The model under review builds one solid part; all positions refer to its coordinate system, in mm. A direction names the side the tool comes from. Coordinates: 2 decimals unless noted, no trailing zeros. Order: outer loops, then holes, each group sorted by start corner. A loop starts at its lowest first (then second) coordinate and runs counter-clockwise, first axis right, second up. Notation, with made-up numbers: M 71.25,13.5 L 95.25,13.5 A30 cw 95.25,46.5 Z; hole C -32.75,37.25 d10. An arc over 180 degrees is marked long. Answer in a Markdown table with one row per item.
Autodesk Inventor part; units mm, degrees
ref_plane "YZ Plane" through (0, 0, 0) normal (1, 0, 0) x (0, 1, 0)
ref_plane "XZ Plane" through (0, 0, 0) normal (0, 1, 0) x (-1, 0, 0)
ref_plane "XY Plane" through (0, 0, 0) normal (0, 0, 1) x (1, 0, 0)
sketch "Sketch1" plane through (0, 0, 0) normal (0, 0, 1) x (1, 0, 0)
  circle A0 centre (0, -12.7) radius 3.175
  circle A1 centre (12.7, 0) radius 3.175
  circle A2 centre (0, 12.7) radius 3.175
  circle A3 centre (-12.7, 0) radius 3.175
  line L0 (25.4, 57.15) -> (-25.4, 57.15)
  line L1 (-25.4, 57.15) -> (-25.4, -57.15)
  line L2 (-25.4, -57.15) -> (25.4, -57.15)
  line L3 (25.4, -57.15) -> (25.4, 57.15)
  point P0 (0, 0)
  dimension "d1" = 6.35
  dimension "d2" = 12.7
  dimension "d5" = 360
  dimension "d13" = 25.4
  dimension "d14" = 57.15
  dimension "d15" = 57.15
  dimension "d16" = 25.4
extrude "Extrusion3" add sketch "Sketch1" along normal blind 6.35
sketch "Sketch3" plane through (0, 0, 6.35) normal (0, 0, 1) x (1, 0, 0)
  line L0 (25.4, 57.15) -> (-25.4, 57.15)
  line L1 (25.4, 57.15) -> (25.4, 50.8)
  line L2 (25.4, -57.15) -> (25.4, 57.15)
  line L3 (25.4, 50.8) -> (-25.4, 50.8)
  line L4 (-25.4, 57.15) -> (-25.4, -57.15)
  line L5 (-25.4, 57.15) -> (25.4, 57.15)
  line L6 (-25.4, -57.15) -> (25.4, -57.15)
  line L7 (25.4, -57.15) -> (25.4, -50.8)
  line L8 (25.4, -50.8) -> (-25.4, -50.8)
  line L9 (-25.4, -50.8) -> (-25.4, -57.15)
  line L10 (-25.4, -57.15) -> (25.4, -57.15)
  point P0 (0, 0)
  dimension "d19" = 6.35
  dimension "d20" = 6.35
extrude "Extrusion4" add sketch "Sketch3" along normal blind 50.8 contours L1 L3 L4 L0 | L2 L6 L4 L8
fillet "Fillet1" radius 3.175 8 edges at (25.4, 53.975, 57.15) (25.4, -53.975, 57.15) (-25.4, -53.975, 57.15) (-25.4, 53.975, 57.15) (0, -57.15, 0) (0, 57.15, 0) (0, -50.8, 6.35) (0, 50.8, 6.35)
sketch "Sketch6" plane through (0, 0, 6.35) normal (0, 0, 1) x (1, 0, 0)
  circle A0 centre (0, 0) radius 3.175
  dimension "d50" = 6.35
extrude "Extrusion6" add sketch "Sketch6" along normal blind 12.7
sketch "Sketch7" plane through (-25.4, 57.15, 3.175) normal (0, 1, 0) x (1, 0, 0)
  line L0 (47.625, -53.975) -> (3.175, -53.975)
  line L1 (0, 0) -> (0, -50.8)
  line L2 (47.625, -53.975) -> (3.175, -53.975)
  line L3 (38.1, -53.975) -> (38.1, -60.325)
  line L4 (12.7, -60.325) -> (12.7, -53.975)
  line L5 (38.1, -60.325) -> (31.75, -60.325)
  line L6 (19.05, -60.325) -> (12.7, -60.325)
  line L7 (38.1, -53.975) -> (12.7, -53.975)
  arc A0 (31.75, -60.325) -> (25.4, -53.975) centre (25.4, -60.325) ccw
  arc A1 (25.4, -53.975) -> (19.05, -60.325) centre (25.4, -60.325) ccw
  point P0 (25.4, 3.175)
  dimension "d57" = 38.1
  dimension "d58" = 12.7
  dimension "d59" = 6.35
  dimension "d60" = 6.35
  dimension "d66" = 6.35
  dimension "d67" = 25.4
  dimension "d68" = 6.35
  dimension "d69" = 25.4
extrude "Extrusion7" add sketch "Sketch7" against normal blind 6.35
sketch "Sketch8" plane through (-25.4, -57.15, 3.175) normal (0, -1, 0) x (1, 0, 0)
  line L0 (12.7, 53.975) -> (12.7, 60.325)
  line L1 (12.7, 53.975) -> (12.7, 60.325)
  line L2 (38.1, 60.325) -> (38.1, 53.975)
  line L3 (38.1, 60.325) -> (38.1, 53.975)
  line L4 (38.1, 53.975) -> (25.4, 53.975)
  line L5 (47.625, 53.975) -> (3.175, 53.975)
  line L6 (12.7, 53.975) -> (25.4, 53.975)
  line L7 (12.7, 60.325) -> (19.05, 60.325)
  line L8 (12.7, 60.325) -> (19.05, 60.325)
  line L9 (31.75, 60.325) -> (38.1, 60.325)
  line L10 (38.1, 60.325) -> (31.75, 60.325)
  arc A0 (19.05, 60.325) -> (25.4, 53.975) centre (25.4, 60.325) ccw
  arc A1 (25.4, 53.975) -> (31.75, 60.325) centre (25.4, 60.325) ccw
  line L11 (0, 0) -> (0, 50.8)
  point P0 (25.4, -3.175)
  dimension "d72" = 6.35
  dimension "d73" = 6.35
  dimension "d74" = 25.4
  dimension "d75" = 25.4
extrude "Extrusion8" add sketch "Sketch8" against normal blind 6.35
sketch "Sketch9" plane through (0, 0, 6.35) normal (0, 0, 1) x (1, 0, 0)
  line L0 (-50.8, 25.4) -> (50.8, 25.4)
  line L1 (50.8, 25.4) -> (50.8, -25.4)
  line L2 (50.8, -25.4) -> (-50.8, -25.4)
  line L3 (-50.8, -25.4) -> (-50.8, 25.4)
  line L4 (-50.8, 25.4) -> (50.8, -25.4) construction
  line L5 (50.8, 25.4) -> (-50.8, -25.4) construction
  line L6 (25.4, -47.625) -> (25.4, 47.625)
  line L7 (25.4, 25.4) -> (25.4, -25.4)
  line L8 (-25.4, 53.975) -> (-25.4, -53.975)
  line L9 (-25.4, 25.4) -> (-25.4, -25.4)
  point P0 (0, 0)
  dimension "d78" = 101.6
  dimension "d79" = 50.8
extrude "Extrusion9" add sketch "Sketch9" against normal blind 6.35 contours L0 L8 L2 L3 | L0 L1 L2 L6
sketch "Sketch11" plane through (0, 0, 6.35) normal (0, 0, 1) x (1, 0, 0)
  line L0 (-25.4, -25.4) -> (-50.8, -25.4)
  line L1 (-50.8, -25.4) -> (-44.45, -25.4)
  line L2 (-44.45, -25.4) -> (-44.45, 25.4)
  line L3 (-25.4, 25.4) -> (-50.8, 25.4)
  line L4 (-50.8, -25.4) -> (-50.8, 25.4)
  line L5 (-50.8, 25.4) -> (-50.8, -25.4)
  line L6 (50.8, -25.4) -> (50.8, 25.4)
  line L7 (50.8, -25.4) -> (50.8, 25.4)
  line L8 (25.4, 25.4) -> (50.8, 25.4)
  line L9 (50.8, 25.4) -> (44.45, 25.4)
  line L10 (44.45, 25.4) -> (44.45, -25.4)
  line L11 (50.8, -25.4) -> (25.4, -25.4)
  line L12 (44.45, -25.4) -> (50.8, -25.4)
  point P0 (0, 0)
  dimension "d84" = 6.35
  dimension "d85" = 6.35
extrude "Extrusion11" add sketch "Sketch11" along normal blind 31.75
fillet "Fillet3" radius 3.175 2 edges at (50.8, 0, 0) (-50.8, 0, 0)
sketch "Sketch18" plane through (0, 0, 38.1) normal (0, 0, 1) x (1, 0, 0)
  line L0 (-50.8, 25.4) -> (-50.8, -25.4)
  line L1 (-50.8, -25.4) -> (50.8, -25.4)
  line L2 (50.8, -25.4) -> (50.8, 25.4)
  line L3 (50.8, 25.4) -> (-50.8, 25.4)
  line L4 (-50.8, 25.4) -> (-50.8, -25.4)
  circle A0 centre (-14.142, -14.142) radius 3.175
  circle A1 centre (14.142, -14.142) radius 3.175
  circle A2 centre (14.142, 14.142) radius 3.175
  circle A3 centre (-14.142, 14.142) radius 3.175
  circle A4 centre (0, 0) radius 3.175
  dimension "d132" = 6.35
  dimension "d137" = 360
  dimension "d139" = 6.35
  dimension "d142" = 14.142
  dimension "d143" = 14.142
extrude "Extrusion16" add sketch "Sketch18" along normal blind 6.35
properties part number "ShoulderPlateXZ"
(1) Take a section at A-A (y = 0). Write out the cut boundary in (x, z) (3 decimals).
Report:
| item | result |
|---|---|
| outline | M -50.8,3.175 A3.175 ccw -47.625,0 L -15.875,0 L -15.875,6.35 L -44.45,6.35 L -44.45,38.1 L -3.175,38.1 L -3.175,44.45 L -50.8,44.45 Z; M -9.525,0 L 9.525,0 L 9.525,6.35 L 3.175,6.35 L 3.175,19.05 L -3.175,19.05 L -3.175,6.35 L -9.525,6.35 Z; M 3.175,38.1 L 44.45,38.1 L 44.45,6.35 L 15.875,6.35 L 15.875,0 L 47.625,0 A3.175 ccw 50.8,3.175 L 50.8,44.45 L 3.175,44.45 Z |
(2) To check wall thickness, follow line 1 (Y direction, x = 0, z = 3.25) (3 decimals); line 2 (Y direction, x = 0, z = 3) (3 decimals); line 3 (Y direction, x = -13.5, z = 48.5). State the ranges of each line that lie inside material, in increasing order. Write a range as [from, to].
Report:
| item | result |
|---|---|
| line 1 | [-57.15, -15.875], [-9.525, 9.525], [15.875, 57.15] |
| line 2 | [-57.145, -15.875], [-9.525, 9.525], [15.875, 57.145] |
| line 3 | [-57.15, -50.8], [50.8, 57.15] |
(3) Take a section at C-C (z = 32). Write out the cut boundary in (x, y), then the cut area to 3 significant figures.
Report:
| item | result |
|---|---|
| outline | M -50.8,-25.4 L -44.45,-25.4 L -44.45,25.4 L -50.8,25.4 Z; M -25.4,-57.15 L 25.4,-57.15 L 25.4,-50.8 L -25.4,-50.8 Z; M -25.4,50.8 L 25.4,50.8 L 25.4,57.15 L -25.4,57.15 Z; M 44.45,-25.4 L 50.8,-25.4 L 50.8,25.4 L 44.45,25.4 Z |
| area | 1,290 mm^2 |
(4) Machinability: for faces 1 (the flat face through (-25.4, -52, 19)), 2 (the flat face through (-18, -54, 57.15)), 3 (the flat face through (0, -50.8, 36)), 4 (the cylindrical face through (17.075, 15.358, 41.231)), 5 (the flat face through (25.4, 52, 19)), which of the approach directions +Z, -Z, +X, -X, +Y, -Y give a long, thin tool a straight path to every point of the face, cutting with its end or side? Answer none if there is none.
Report:
| item | result |
|---|---|
| face 1 | +Z, -Z, -X, -Y |
| face 2 | +Z, -X, +Y, -Y |
| face 3 | +Z, +X, -X |
| face 4 | +Z |
| face 5 | +Z, -Z, +X, +Y |
(5) Take a section at B-B (x = 8). Write out the cut boundary in (y, z) (3 decimals), then the cut area to 3 significant figures.
Report:
| item | result |
|---|---|
| outline | M -57.15,3.175 A3.175 ccw -53.975,0 L 53.975,0 A3.175 ccw 57.15,3.175 L 57.15,63.5 L 50.8,63.5 L 50.8,9.525 A3.175 cw 47.625,6.35 L -47.625,6.35 A3.175 cw -50.8,9.525 L -50.8,63.5 L -57.15,63.5 Z; M -25.4,38.1 L 25.4,38.1 L 25.4,44.45 L -25.4,44.45 Z |
| area | 1,770 mm^2 |
(6) Insertion check: P1, Ø1.9, axis at y = 52.5, z = 60, coming from the +X side; P2, Ø12, axis at x = -27.5, y = 34.5, coming from the +Z side; P3, Ø1.9, axis at x = 16.5, y = -55, coming from the +Z side. Each pin has a flat end and moves straight along its axis. Give the tip position at first contact, or say it passes through.
Report:
| item | result |
|---|---|
| P1 | x = 12.7 |
| P2 | z = 6.35 |
| P3 | z = 57.15 |
(7) Take a section at D-D (x = 43). Write out the cut boundary in (y, z), then the cut area to 3 significant figures.
Report:
| item | result |
|---|---|
| outline | M -25.4,0 L 25.4,0 L 25.4,6.35 L -25.4,6.35 Z; M -25.4,38.1 L 25.4,38.1 L 25.4,44.45 L -25.4,44.45 Z |
| area | 645 mm^2 |
(8) The part is to be moulded in two halves that separate along Z. For faces 6 (the flat face through (-25.4, 52, 19)), 7 (the cylindrical face through (-0.69, 3.1, 12.61)), 8 (the flat face through (-1, 1, 0)), 9 (the cylindrical face through (24.49, 53.93, 56.2)), say which applies: +Z half, -Z half, draft (parallel to the pull), parting line (faces both ways), or undercut.
Report:
| item | result |
|---|---|
| face 6 | draft |
| face 7 | undercut |
| face 8 | -Z half |
| face 9 | +Z half |
